Geometry: final body of the model. Coordinates: model frame, mm. A direction names the side the tool comes from. Round coordinates to 2 decimals unless told otherwise and drop trailing zeros. Write each loop counter-clockwise with the first axis right and the second up, starting at its lowest first coordinate (ties: lowest second). Pieces come first, ordered by that corner, then holes. Notation, with made-up numbers: (-36, 63) - (-13, 63) arc R27 cw to (-13, 90) - close; hole circle Ø3 at (-17, 65). An arc over 180 degrees is marked (long way). Use a Markdown table: item, result. Add a question column.
```python
from build123d import *

# Parameters (mm, degrees)
F0_W     = 3.175
F0_H     = 25.4
F1_DEPTH = 1219.2
F3_D     = 8.4328


with BuildPart() as f1:
    # F0 (on Front) → F1 (new body)
    with BuildSketch(Plane.XZ):
        with Locations((-17.4625, 14.2875)):
            Rectangle(F0_W, F0_H)
        with Locations((17.4625, 14.2875)):
            Rectangle(F0_W, F0_H)
        Polygon((-19.05, -1.5875), (19.05, -1.5875), (19.05, 1.5875), (15.875, 1.5875), (-15.875, 1.5875), (-19.05, 1.5875), align=None)
    extrude(amount=F1_DEPTH)

    # F3 (through all)
    with Locations(Plane.XY.offset(1.5875)):
        with Locations((0, -26.2155216187), (0, -80.6770920753), (0, -140.1309669018), (0, -202.7617692947)):
            Hole(F3_D / 2)


solid = f1.part
```
1) Material intervals for L1, parallel to Y at x = 0, z = 0.7; L2, parallel to X at y = -344.5, z = 18.75 (3 decimals); L3, parallel to Z at x = -4, y = -609, sorted ascending. Write a range as from..to.
2) Pin query (flat end, axial travel): P1, Ø12, axis at x = 0, y = -179.5, coming from the +Z side. Return the tip coordinate at first contact, or that it passes through.
3) Set-up query: faces 1 (the flat face through (1, 0, 1)), 2 (the flat face through (-15.875, -601, 14)). Return all of +Z, -Z, +X, -X, +Y, -Y with unobstructed straight access to the full face (end or side cutting, diameter ignored); none if empty.
4) Section B-B, the plane x = -10. Return the cut outline in (y, z).
5) Draft query along X for faces 3 (the flat face through (-19.05, -601, 13)), 4 (the flat face through (0, -601, -1.588)), 5 (the flat face through (0, -601, 1.588)), 6 (the flat face through (19.05, -601, 12)). Return one class per face: released by +X, released by -X, zero draft, split by the parting line, or undercut.
Output values:
| question | item | result |
|---|---|---|
| 1 | L1 | y = -1219.2..-206.98, -198.55..-144.35, -135.91..-84.89, -76.46..-30.43, -22..0 |
| 1 | L2 | x = -19.05..-15.875, 15.875..19.05 |
| 1 | L3 | z = -1.59..1.59 |
| 2 | P1 | stops at z = 1.59 |
| 3 | face 1 | +Z, -Z, +X, -X, +Y |
| 3 | face 2 | +Z, +Y, -Y |
| 4 | outline | (-1219.2, -1.59) - (0, -1.59) - (0, 1.59) - (-1219.2, 1.59) - close |
| 5 | face 3 | released by -X |
| 5 | face 4 | zero draft |
| 5 | face 5 | undercut |
| 5 | face 6 | released by +X |
